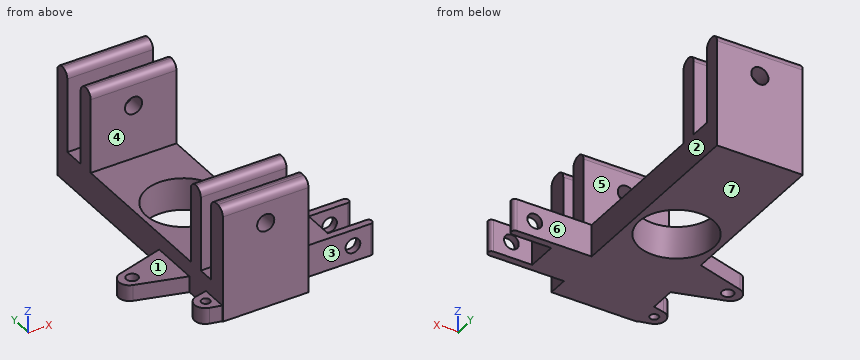
```python
from build123d import *

# Parameters (mm, degrees)
SKETCH2_W               = 80
SKETCH2_H               = 248
BOSS_EXTRUDE1_DEPTH     = 30
BOSS_EXTRUDE2_DEPTH     = 15
SKETCH3_W               = 80
SKETCH3_H               = 15
SKETCH3_W_2             = 79.927982428
SKETCH3_H_2             = 17.63
BOSS_EXTRUDE3_DEPTH     = 107
FILLET1_R               = 7.5
FILLET2_R               = 3.33
CUT_EXTRUDE1_DEPTH      = 311.421758238
CUT_EXTRUDE1_DEPTH_BACK = 311.421758238
SKETCH4_R               = 35
CUT_EXTRUDE2_DEPTH      = 311.421758238
CUT_EXTRUDE2_DEPTH_BACK = 311.421758238
SKETCH5_R               = 8
SKETCH6_R               = 6.855911781
CUT_EXTRUDE3_DEPTH      = 265.72901312
SKETCH7_R               = 5.441513082
CUT_EXTRUDE4_DEPTH      = 306.575961076
SKETCH8_R               = 4
CUT_EXTRUDE5_DEPTH      = 306.575961076


# Some blends are built 0.0001 mm under size
with BuildPart() as part:
    # Sketch2 → Boss-Extrude1 (new body)
    with BuildSketch(Plane.XY):
        with Locations((40, 124)):
            Rectangle(SKETCH2_W, SKETCH2_H)
        Polygon((153, 60.32), (80, 60.32), (80, 18.794599866), (153, 18.794599866), (153, 25.284599866), (113.63, 25.284599866), (113.63, 53.83), (153, 53.83), align=None)
    extrude(amount=BOSS_EXTRUDE1_DEPTH)

    # Sketch2<5> → Boss-Extrude2 (add)
    with BuildSketch(Plane.XY):
        with BuildLine():
            Line((0, 50), (0, 95.32))
            Line((0, 95.32), (-44.67244089, 82.258125951))
            ThreePointArc((-44.67244089, 82.258125951), (-51.866023561, 72.66), (-44.67244089, 63.061874049))
            Line((-44.67244089, 63.061874049), (0, 50))
        make_face()
        with BuildLine():
            Line((-10.531496207, 3.314319271), (0, 0.795400134))
            Line((0, 0.795400134), (0, 25.284599866))
            Line((0, 25.284599866), (-10.531496207, 22.765680729))
            ThreePointArc((-10.531496207, 22.765680729), (-18.205311701, 13.04), (-10.531496207, 3.314319271))
        make_face()
    extrude(amount=BOSS_EXTRUDE2_DEPTH)

    # Sketch3 → Boss-Extrude3 (add)
    with BuildSketch(Plane.XY):
        with Locations((40, 240.5)):
            Rectangle(SKETCH3_W, SKETCH3_H)
        with Locations((40, 205.5)):
            Rectangle(SKETCH3_W, SKETCH3_H)
        with Locations((40, 40.5)):
            Rectangle(SKETCH3_W, SKETCH3_H)
        with Locations((39.963991214, 8.815)):
            Rectangle(SKETCH3_W_2, SKETCH3_H_2)
    extrude(amount=BOSS_EXTRUDE3_DEPTH)

    # Fillet1
    fillet1_edges = [part.edges().sort_by_distance(p)[0] for p in [
        (39.963991214, 0, 107),
        (39.963991214, 17.63, 107),
        (40, 33, 107),
        (40, 48, 107),
        (40, 198, 107),
        (40, 213, 107),
        (40, 233, 107),
        (40, 248, 107),
    ]]
    fillet(fillet1_edges, radius=FILLET1_R - 0.0001)  # a hair under: the kernel refuses the full size

    # Fillet2
    # the kernel refuses this fillet: 3.33 mm, written as the material it takes off along each edge
    with BuildSketch(Plane(origin=(153, 18.794599866, -8.325), x_dir=(-1, 0, 0), z_dir=(0, 0, 1)), Plane(origin=(153, 25.284599866, -8.325), x_dir=(0, -1, 0), z_dir=(0, 0, 1)), Plane(origin=(153, 53.83, -8.325), x_dir=(-1, 0, 0), z_dir=(0, 0, 1)), Plane(origin=(153, 60.32, -8.325), x_dir=(0, -1, 0), z_dir=(0, 0, 1))) as fillet2_piece_1:
        with BuildLine():
            CenterArc((FILLET2_R, -FILLET2_R), FILLET2_R, 90, 90)
            Line((0, -FILLET2_R), (0, 0))
            Line((0, 0), (FILLET2_R, 0))
        make_face()
    extrude(amount=46.65, mode=Mode.SUBTRACT)

    # Sketch4 → Cut-Extrude1 (cut, two sides: drawn at the far end of the back side and taken through both)
    with BuildSketch(Plane.XY.offset(-CUT_EXTRUDE1_DEPTH_BACK)):
        with Locations((39.848575035, 123)):
            Circle(SKETCH4_R)
    extrude(amount=CUT_EXTRUDE1_DEPTH + CUT_EXTRUDE1_DEPTH_BACK, mode=Mode.SUBTRACT)

    # Sketch5 → Cut-Extrude2 (cut, two sides: drawn at the far end of the back side and taken through both)
    with BuildSketch(Plane(origin=(0, 0, 0), x_dir=(1, 0, 0), z_dir=(0, 1, 0)).offset(-CUT_EXTRUDE2_DEPTH_BACK)):
        with Locations(Location((40, -80, 0), (0, 0, 270))):
            Circle(SKETCH5_R)
    extrude(amount=CUT_EXTRUDE2_DEPTH + CUT_EXTRUDE2_DEPTH_BACK, mode=Mode.SUBTRACT)

    # Sketch6 → Cut-Extrude3 (cut, through all)
    with BuildSketch(Plane(origin=(0, 60.32, 0), x_dir=(1, 0, 0), z_dir=(0, 1, 0))):
        with Locations(Location((133.07, -15, 0), (0, 0, 270))):
            Circle(SKETCH6_R)
    extrude(amount=-CUT_EXTRUDE3_DEPTH, mode=Mode.SUBTRACT)

    # Sketch7 → Cut-Extrude4 (cut, through all)
    with BuildSketch(Plane.XY.offset(15)):
        with Locations((-39.33, 72.66)):
            Circle(SKETCH7_R)
    extrude(amount=-CUT_EXTRUDE4_DEPTH, mode=Mode.SUBTRACT)

    # Sketch8 → Cut-Extrude5 (cut, through all)
    with BuildSketch(Plane.XY.offset(15)):
        with Locations((-7.83, 13.04)):
            Circle(SKETCH8_R)
    extrude(amount=-CUT_EXTRUDE5_DEPTH, mode=Mode.SUBTRACT)


solid = part.part
```
Geometry: final body of the model. Coordinates: model frame, mm. Face numbers are marked on the shaded views. A direction names the side the tool comes from. Coordinates: 2 decimals unless noted, no trailing zeros. Order: outer loops, then holes, each group sorted by start corner. A loop starts at its lowest first (then second) coordinate and runs counter-clockwise, first axis right, second up. Notation, with made-up numbers: (38.5, -39) - (94.5, -39) arc R27 ccw to (94.5, -18) - close; hole circle Ø1 at (65.25, -10.5). An arc over 180 degrees is marked (long way). Return JSON: item names as keys, results as strings. Group by question number.
1. Cut plane D-D (y = 13.04). Output: boundary loops of the cut face in (x, z), plus the area to 3 significant figures.
2. Cut plane A-A (y = 123). Output: boundary loops of the cut face in (x, z), plus the area to 3 significant figures.
3. Set-up query: the marked faces 1, 2, 3 and 4. Return all of +Z, -Z, +X, -X, +Y, -Y with unobstructed straight access to the full face (end or side cutting, diameter ignored); none if empty.
4. Material intervals for line 1 along Y through (x, z) = (26, 32.5); line 2 along X through (y, z) = (13, 9); line 3 along X through (y, z) = (239, 80), sorted ascending. Write a range as [from, to].
5. Pull-direction query (Y, two-part tool) for the marked faces 5, 6 and 7; classes: pulls with the +Y half, pulls with the -Y half, needs draft (parallel to the pull), parting line crosses it, or undercut.
6. Cut plane B-B (z = 65). Output: boundary loops of the cut face in (x, y).
7. Pin query (flat end, axial travel): pin 1 (4.5 mm diameter, centred on y = 42, z = 78, fed in from +X); pin 2 (4 mm diameter, centred on y = 126.5, z = 22, fed in from -X); pin 3 (24 mm diameter, centred on x = 131.5, z = 12.5, fed in from -Y). Return the tip coordinate at first contact, or that it passes through.
Resolved:
{
 "1": {"outline": "(-18.21, 0) - (-11.83, 0) - (-11.83, 15) - (-18.21, 15) - close; (-3.83, 0) - (80, 0) - (80, 30) - (79.93, 30) - (79.93, 106.41) - (0, 106.41) - (0, 15) - (-3.83, 15) - close; hole circle Ø16 at (40, 80)", "area": "8,460 mm²"},
 "2": {"outline": "(0, 0) - (4.85, 0) - (4.85, 30) - (0, 30) - close; (74.85, 0) - (80, 0) - (80, 30) - (74.85, 30) - close", "area": "300 mm²"},
 "3": {"face 1": "+Z, -X, +Y, -Y", "face 2": "+Z, -Z, +X, +Y", "face 3": "+Z, -Z, +X, -Y", "face 4": "+Z, +X, -X"},
 "4": {"line 1": "y = [0, 17.63], [33, 48], [198, 213], [233, 248]", "line 2": "x = [-18.21, -11.83], [-3.83, 80]", "line 3": "x = [0, 32], [48, 80]"},
 "5": {"face 5": "undercut", "face 6": "pulls with the +Y half", "face 7": "needs draft"},
 "6": {"outline": "(0, 0) - (79.93, 0) - (79.93, 17.63) - (0, 17.63) - close; (0, 33) - (80, 33) - (80, 48) - (0, 48) - close; (0, 198) - (80, 198) - (80, 213) - (0, 213) - close; (0, 233) - (80, 233) - (80, 248) - (0, 248) - close"},
 "7": {"pin 1": "stops at x = 80", "pin 2": "stops at x = 0", "pin 3": "stops at y = 18.79"}
}
